Autodesk Fusion 360 part; units mm, degrees
sketch "Sketch1" plane through (0, 0, 0) normal (0, 1, 0) x (1, 0, 0)
  line L0 (609.6, 0) -> (609.6, 609.6)
  line L1 (0, 609.6) -> (0, 0)
  line L2 (0, 0) -> (88.9, 0)
  line L3 (88.9, 609.6) -> (0, 609.6)
  line L4 (0, 609.6) -> (0, 0)
  line L5 (609.6, 609.6) -> (520.7, 609.6)
  line L6 (520.7, -460.804) -> (609.6, -460.804)
  line L7 (609.6, -460.804) -> (609.6, 609.6)
  line L8 (609.6, 304.8) -> (609.6, 355.6)
  line L9 (520.7, 355.6) -> (88.9, 355.6)
  line L10 (0, 355.6) -> (0, 304.8)
  line L11 (609.6, 304.8) -> (609.6, 254)
  line L12 (520.7, 254) -> (88.9, 254)
  line L13 (0, 254) -> (0, 304.8)
  line L14 (88.9, 0) -> (88.9, 254)
  line L15 (88.9, 355.6) -> (88.9, 609.6)
  line L16 (520.7, 609.6) -> (520.7, 355.6)
  line L17 (520.7, 254) -> (520.7, 0)
  line L18 (0, 0) -> (88.9, 0)
  line L19 (520.7, 0) -> (609.6, 0)
  line L20 (609.6, 609.6) -> (520.7, 609.6)
  line L21 (88.9, 609.6) -> (0, 609.6)
  dimension "d1" = 609.6
  dimension "d2" = 609.6
  dimension "d3" = 88.9
  dimension "d4" = 88.9
  dimension "d5" = 50.8
  dimension "d6" = 50.8
extrude "Extrude1" add sketch "Sketch1" along normal blind 25.4
sketch "Sketch2" plane through (0, 0, 0) normal (0, -1, 0) x (1, 0, 0)
  line L0 (609.6, -609.6) -> (609.6, 0)
  line L1 (609.6, 0) -> (520.7, 0)
  line L2 (520.7, 0) -> (520.7, -254)
  line L3 (520.7, -254) -> (88.9, -254)
  line L4 (88.9, -254) -> (88.9, 0)
  line L5 (88.9, 0) -> (0, 0)
  line L6 (0, 0) -> (0, -609.6)
  line L7 (0, -609.6) -> (88.9, -609.6)
  line L8 (88.9, -609.6) -> (88.9, -355.6)
  line L9 (88.9, -355.6) -> (520.7, -355.6)
  line L10 (520.7, -355.6) -> (520.7, -609.6)
  line L11 (520.7, -609.6) -> (609.6, -609.6)
  line L12 (0, 0) -> (88.9, 0)
  line L13 (88.9, 0) -> (88.9, -609.6)
  line L14 (88.9, -609.6) -> (0, -609.6)
  line L15 (0, -609.6) -> (0, 0)
  line L16 (520.7, 0) -> (609.6, 0)
  line L17 (609.6, 0) -> (609.6, -609.6)
  line L18 (609.6, -609.6) -> (520.7, -609.6)
  line L19 (520.7, -609.6) -> (520.7, 0)
extrude "Extrude2" add sketch "Sketch2" along normal blind 63.5 contours L0 L1 L2 L10 L11 L16 L17 L18 L19 | L4 L5 L6 L7 L8 L12 L13 L14 L15
sketch "Sketch3" plane through (0, 25.4, 0) normal (0, 1, 0) x (-1, 0, 0)
  line L0 (-609.6, 0) -> (-609.6, -609.6)
  line L1 (-609.6, -609.6) -> (-520.7, -609.6)
  line L2 (-520.7, -609.6) -> (-520.7, -355.6)
  line L3 (-520.7, -355.6) -> (-88.9, -355.6)
  line L4 (-88.9, -355.6) -> (-88.9, -609.6)
  line L5 (-88.9, -609.6) -> (0, -609.6)
  line L6 (0, -609.6) -> (0, 0)
  line L7 (0, 0) -> (-88.9, 0)
  line L8 (-88.9, 0) -> (-88.9, -254)
  line L9 (-88.9, -254) -> (-520.7, -254)
  line L10 (-520.7, -254) -> (-520.7, 0)
  line L11 (-520.7, 0) -> (-609.6, 0)
  circle A0 centre (-304.8, -304.8) radius 50.8
extrude "Extrude3" add sketch "Sketch3" along normal blind 762 contours A0
extrude "Extrude4" cut 1 faces at (289.3545, 787.4, -299.9767) along direction (0, -1, 0) blind 101.6
sketch "Sketch4" plane through (0, -63.5, 0) normal (0, -1, 0) x (1, 0, 0)
  line L0 (0, -609.6) -> (88.9, -609.6)
  line L1 (88.9, -609.6) -> (88.9, 0)
  line L2 (88.9, 0) -> (0, 0)
  line L3 (0, 0) -> (0, -609.6)
  line L4 (44.45, 0) -> (44.45, -609.6)
  line L5 (44.45, 0) -> (44.45, -11.9009)
  line L6 (44.45, 0) -> (44.45, -76.2)
  line L7 (44.45, -609.6) -> (44.45, -533.4)
  dimension "d15" = 76.2
  dimension "d16" = 76.2
sphere "SpherePrimitive1" add diameter 50.8 placed x (1, 0, 0) y (0, 0, 1) z (0, -1, 0) at (44.23, -63.5, -74.8157)
sphere "SpherePrimitive2" add diameter 50.8 placed x (1, 0, 0) y (0, 0, 1) z (0, -1, 0) at (44.8206, -63.5, -533.484)
sketch "Sketch7" plane through (0, -63.5, 0) normal (0, -1, 0) x (1, 0, 0)
  line L0 (520.7, -609.6) -> (609.6, -609.6)
  line L1 (609.6, -609.6) -> (609.6, 0)
  line L2 (609.6, 0) -> (520.7, 0)
  line L3 (520.7, 0) -> (520.7, -609.6)
  line L4 (565.15, 0) -> (565.15, -609.6)
  line L5 (565.15, 0) -> (565.15, -76.2)
  line L6 (565.15, -609.6) -> (565.15, -533.4)
  dimension "d19" = 76.2
  dimension "d20" = 76.2
sphere "SpherePrimitive3" add diameter 50.8 placed x (1, 0, 0) y (0, 0, 1) z (0, -1, 0) at (565.3152, -63.5, -75.9261)
sphere "SpherePrimitive4" add diameter 50.8 placed x (1, 0, 0) y (0, 0, 1) z (0, -1, 0) at (565.1233, -63.5, -532.8086)
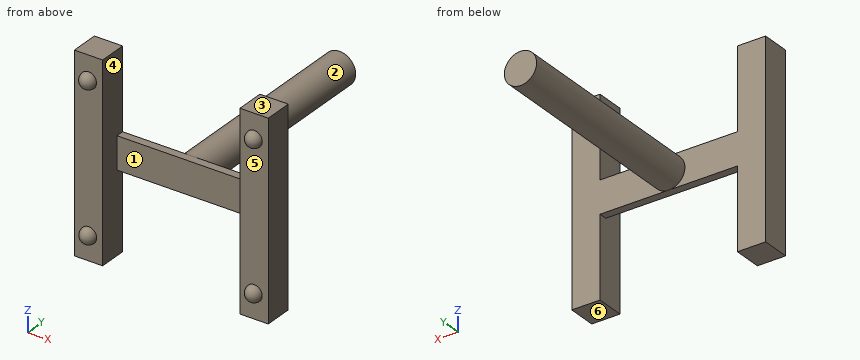
Can you work these out from the model? Positions are in its coordinate system, mm. Face numbers are marked on the shaded views. A direction names the side the tool comes from. Round coordinates to 2 decimals unless told otherwise and drop trailing zeros. Loops run counter-clockwise (first coordinate to the right, second up) from the corner with the lowest first, then second, coordinate; pieces in that order, holes last.
Item 1: Suppose I cut it at C-C, the plane x = 325. Write out the boundary of the cut face in (y, z), then the cut area to 3 significant figures.
Item 2: Please list where these lines run through material, in increasing order: L1, parallel to X at y = -43, z = -391; L2, parallel to Y at x = 143.5, z = -313.5; L3, parallel to Y at x = 69.5, z = -113.
Item 3: If we mould it in two halves opening along Z, with no side actions, what happens to the marked faces 4, 5 and 6? For each: +Z half, -Z half, draft (parallel to the pull), parting line (faces both ways), or undercut.
Item 4: Will these pins go through, and if not, where does the flat tip stop? pin 1 Ø1.5 at (y, z) = (314.5, -339) entering from +X; pin 2 Ø7.5 at (x, y) = (222, 10.5) entering from +Z; pin 3 Ø12 at (y, z) = (273, -363.5) entering from +X; pin 4 Ø8 at (x, z) = (192, -259.5) entering from +Y.
Item 5: Suppose I cut it at D-D, the plane y = 201.5. Write out the boundary of the cut face in (x, z).
Item 6: Suppose I cut it at B-B, the plane z = -304.8. Write out the boundary of the cut face in (x, y), then the cut area to 3 significant figures.
Item 7: Suppose I cut it at A-A, the plane z = -154. Write out the boundary of the cut face in (x, y), then the cut area to 3 significant figures.
Item 8: Which directions (+Z, -Z, +X, -X, +Y, -Y) give clear straight access to the entire face, cutting with the end or side of a thin tool? Please do the marked faces 1, 2 and 3.
Reported:
1. outline: (0, -355.6) - (25.4, -355.6) - (25.4, -351.41) - (685.8, -351.41) - (685.8, -258.19) - (25.4, -258.19) - (25.4, -254) - (0, -254) - close
1. area: 64,100 mm2
2. L1: x = 0 to 88.9, 520.7 to 609.6
2. L2: y = 0 to 25.4
2. L3: y = -63.5 to 25.4
3. face 4: draft
3. face 5: undercut
3. face 6: -Z half
4. pin 1: stops at x = 343.03
4. pin 2: stops at z = -254
4. pin 3: passes through
4. pin 4: stops at y = 25.4
5. outline: circle Ø101.6 at (304.8, -304.8)
6. outline: (0, -63.5) - (88.9, -63.5) - (88.9, 0) - (520.7, 0) - (520.7, -63.5) - (609.6, -63.5) - (609.6, 25.4) - (355.6, 25.4) - (355.6, 685.8) - (254, 685.8) - (254, 25.4) - (0, 25.4) - close
6. area: 93,900 mm2
7. outline: (0, -63.5) - (88.9, -63.5) - (88.9, 25.4) - (0, 25.4) - close; (520.7, -63.5) - (609.6, -63.5) - (609.6, 25.4) - (520.7, 25.4) - close
7. area: 15,800 mm2
8. face 1: +Z, -Z, -Y
8. face 2: +Y
8. face 3: +Z, +X, -X, +Y, -Y
